Source: CAD feature listing. Evaluate the final solid. Frame: model axes, mm. Face numbers are marked on the shaded views. A direction names the side the tool comes from. Coordinates: 2 decimals unless noted, no trailing zeros. Loops run counter-clockwise (first coordinate to the right, second up) from the corner with the lowest first, then second, coordinate; pieces in that order, holes last. Notation, with made-up numbers: (53.25, 19) - (80.25, 19) arc R32 ccw to (80.25, 53) - close; hole circle Ø6 at (-11, 74). An arc over 180 degrees is marked (long way). Use CSV: the item, a comma, the result in double quotes. Start each with the question number.
```python
from build123d import *

# Parameters (mm, degrees)
F0_R     = 8.509
F1_DEPTH = 5.08
F2_R     = 7.1501
F3_DEPTH = 8.636
F5_D     = 7.9375
F6_SIZE2 = 1.524
F6_SIZE  = 1.524


with BuildPart() as f1:
    # F0 (on Top) → F1 (new body)
    with BuildSketch(Plane.XY):
        Circle(F0_R)
    extrude(amount=F1_DEPTH)

    # F2 (on face) → F3 (join)
    with BuildSketch(Plane.XY.offset(5.08)):
        Circle(F2_R)
    extrude(amount=F3_DEPTH)

    # F5 (through all)
    with Locations(Plane(origin=(0, 0, 0), x_dir=(1, 0, 0), z_dir=(0, 0, -1))):
        with Locations((0, 0)):
            Hole(F5_D / 2)

    # F6
    f6_edges = [f1.edges().sort_by_distance(p)[0] for p in [
        (-8.509, 0, 0),
    ]]
    chamfer(f6_edges, length=F6_SIZE, length2=F6_SIZE2)


solid = f1.part
```
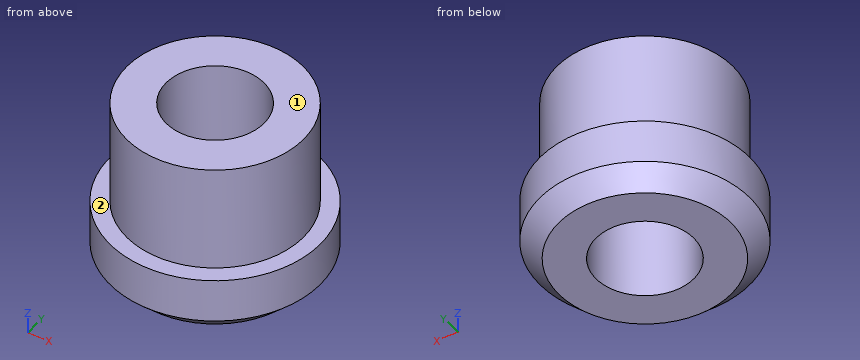
(1) Section C-C on z = 11.5. Output: boundary loops of the cut face in (x, y), plus the area to 3 significant figures.
(2) Pin query (flat end, axial travel): pin 1 Ø4 at (x, z) = (-6, 4) entering from -Y; pin 2 Ø8 at (y, z) = (-1, 11) entering from -X; pin 3 Ø6 at (y, z) = (-5, 10) entering from +X. Return the tip coordinate at first contact, or that it passes through.
(3) Section A-A on x = 0. Output: boundary loops of the cut face in (y, z) (3 decimals).
(4) Ray query, line 1 (Y direction, x = 0, z = 8.5); line 2 (Y direction, x = 0, z = 4.75); line 3 (X direction, y = 2.75, z = 10). Return the intervals inside material, ascending. Write a range as [from, to].
(5) Reachability of the marked faces 1 and 2 from +Z, -Z, +X, -X, +Y, -Y: full face, straight path, thin tool, end or side. Return the list, or none.
Solution:
1,outline,"circle Ø14.3 at (0, 0); hole circle Ø7.94 at (0, 0)"
1,area,"111 mm²"
2,pin 1,"stops at y = -7.51"
2,pin 2,"stops at x = -7.15"
2,pin 3,"stops at x = 6.86"
3,outline,"(-8.509, 1.524) - (-6.985, 0) - (-3.969, 0) - (-3.969, 13.716) - (-7.15, 13.716) - (-7.15, 5.08) - (-8.509, 5.08) - close; (3.969, 0) - (6.985, 0) - (8.509, 1.524) - (8.509, 5.08) - (7.15, 5.08) - (7.15, 13.716) - (3.969, 13.716) - close"
4,line 1,"y = [-7.15, -3.97], [3.97, 7.15]"
4,line 2,"y = [-8.51, -3.97], [3.97, 8.51]"
4,line 3,"x = [-6.6, -2.86], [2.86, 6.6]"
5,face 1,"+Z, +X, -X, +Y, -Y"
5,face 2,"+Z"
